Input: dimensioned drawing with shaded views. Units: mm. Origin: part minimum x, y, z. Round coordinates to 2 decimals unless told otherwise and drop trailing zeros. Order: outer loops, then holes, each group sorted by start corner. A loop starts at its lowest first (then second) coordinate and runs counter-clockwise, first axis right, second up. Notation, with made-up numbers: (-20.5, 17.5) - (7.5, 17.5) arc R10 ccw to (7.5, 22.5) - close; hole circle Ø10 at (24.5, -24). An arc over 180 degrees is marked (long way). Put each result on its own line as item: value. Start each with the question number.
(1) Pin query (flat end, axial travel): P1, Ø4, axis at x = 2, y = 35, coming from the +Z side; P2, Ø6, axis at x = 6.5, y = 41.5, coming from the -Z side; P3, Ø3, axis at x = 2, y = 6.5, coming from the +Z side; P4, Ø1.1, axis at y = 1.5, z = 23, coming from the -X side. Return the tip coordinate at first contact, or that it passes through.
(2) Material intervals for L1, parallel to Y at x = 5.5, z = 8.95; L2, parallel to Z at x = 6.25, y = 26; L3, parallel to X at y = 47, z = 8.5, sorted ascending. Write a range as [from, to].
(3) Section C-C (y = 16). Output: boundary loops of the cut face in (x, z), and give its area (3 significant figures).
(4) Section A-A (x = 7.25). Output: boundary loops of the cut face in (y, z) (1 decimal), and give its area (3 significant figures).
(5) Pull-direction query (Y, two-part tool) for the marked faces 1, 2, 3 and 4; classes: released by +Y, released by -Y, zero draft, split by the parting line, or undercut.
(6) Section B-B (z = 15.5). Output: boundary loops of the cut face in (x, y).
(7) Section D-D (z = 10.5). Output: boundary loops of the cut face in (x, y).
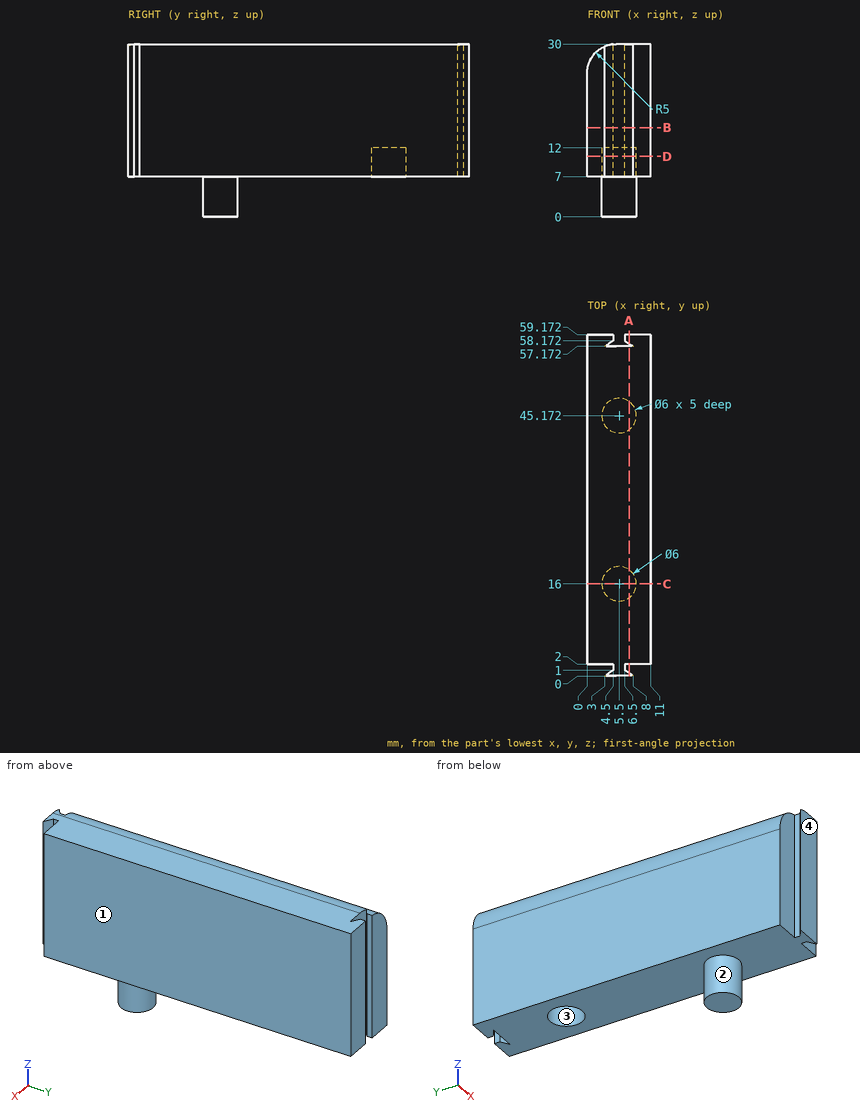
Checks:
1. P1: stops at z = 29.9
1. P2: stops at z = 7
1. P3: stops at z = 29.77
1. P4: stops at x = 0
2. L1: y = [0, 42.17], [48.17, 57.17]
2. L2: z = [7, 30]
2. L3: x = [0, 3.12], [7.88, 11]
3. outline: (0, 7) - (2.5, 7) - (2.5, 0) - (8.5, 0) - (8.5, 7) - (11, 7) - (11, 30) - (5, 30) arc R5 ccw to (0, 25) - close
3. area: 290 mm²
4. outline: (0, 7) - (0.5, 7) - (0.5, 30) - (0, 30) - close; (2, 7) - (13.6, 7) - (13.6, 0) - (18.4, 0) - (18.4, 7) - (42.7, 7) - (42.7, 12) - (47.6, 12) - (47.6, 7) - (57.2, 7) - (57.2, 30) - (2, 30) - close; (57.7, 7) - (59.2, 7) - (59.2, 30) - (57.7, 30) - close
4. area: 1,320 mm²
5. face 1: zero draft
5. face 2: split by the parting line
5. face 3: undercut
5. face 4: released by -Y
6. outline: (0, 2) - (4.5, 2) - (4.5, 1) - (3, 0) - (8, 0) - (6.5, 1) - (6.5, 2) - (11, 2) - (11, 59.17) - (6.5, 59.17) - (6.5, 58.17) - (8, 57.17) - (3, 57.17) - (4.5, 58.17) - (4.5, 59.17) - (0, 59.17) - close
7. outline: (0, 2) - (4.5, 2) - (4.5, 1) - (3, 0) - (8, 0) - (6.5, 1) - (6.5, 2) - (11, 2) - (11, 59.17) - (6.5, 59.17) - (6.5, 58.17) - (8, 57.17) - (3, 57.17) - (4.5, 58.17) - (4.5, 59.17) - (0, 59.17) - close; hole circle Ø6 at (5.5, 45.17)
